Geometry: final body of the model. Coordinates: model frame, mm. A direction names the side the tool comes from. Round coordinates to 2 decimals unless told otherwise and drop trailing zeros. Loops run counter-clockwise (first coordinate to the right, second up) from the corner with the lowest first, then second, coordinate; pieces in that order, holes last. Notation, with made-up numbers: M -27,84.5 L 2,84.5 A11 cw 2,93.5 Z; hole C 49,73 d3. An arc over 180 degrees is marked long. Answer as a JSON object with one key per item and string values.
from build123d import *

# Parameters (mm, degrees)
F0_W     = 50.8
F0_H     = 76.2
F1_DEPTH = 101.6
F2_R     = 3.175
F3_W     = 6.770242
F3_H     = 4.11195
F4_DEPTH = 152.4


with BuildPart() as f1:
    # F0 (on Front) → F1 (new body)
    with BuildSketch(Plane.XZ):
        with Locations((25.4, 38.1)):
            Rectangle(F0_W, F0_H)
    extrude(amount=F1_DEPTH)

    # F2
    f2_edges = [f1.edges().sort_by_distance(p)[0] for p in [
        (50.8, -50.8, 76.2),
        (0, -50.8, 76.2),
        (25.4, 0, 76.2),
        (25.4, -101.6, 76.2),
        (0, -50.8, 0),
        (50.8, -50.8, 0),
        (25.4, 0, 0),
        (25.4, -101.6, 0),
    ]]
    fillet(f2_edges, radius=F2_R)

    # F3 (on face) → F4 (join)
    with BuildSketch(Plane.XY.offset(76.2)):
        with Locations((28.007837, -26.172377)):
            Rectangle(F3_W, F3_H)
    extrude(amount=F4_DEPTH)


solid = f1.part
1) Reachability of faces 1 (the flat face through (31.393, -26, 151)), 2 (the flat face through (28, -24.116, 151)), 3 (the flat face through (28, -28.228, 151)), 4 (the flat face through (24.623, -26, 151)) from +Z, -Z, +X, -X, +Y, -Y: full face, straight path, thin tool, end or side. Return the list, or none.
Results:
{"face 1": "+Z, +X, +Y, -Y", "face 2": "+Z, +X, -X, +Y", "face 3": "+Z, +X, -X, -Y", "face 4": "+Z, -X, +Y, -Y"}
2) Section query B-B (x = 15). Return the cut outline in (y, z) (3 decimals).
Results:
{"outline": "M -101.6,3.175 A3.175 ccw -98.425,0 L -3.175,0 A3.175 ccw 0,3.175 L 0,73.025 A3.175 ccw -3.175,76.2 L -98.425,76.2 A3.175 ccw -101.6,73.025 Z"}
3) Section query C-C (z = 142). Return the cut outline in (x, y), and give its area (3 significant figures).
Results:
{"outline": "M 24.62,-28.23 L 31.39,-28.23 L 31.39,-24.12 L 24.62,-24.12 Z", "area": "27.8 mm2"}
4) Ray query, line 1 (Z direction, x = 8.5, y = -95.5); line 2 (Y direction, x = 30.5, z = 84); line 3 (X direction, y = -54, z = 73.5). Return the intervals inside material, ascending.
Results:
{"line 1": "0 to 76.2", "line 2": "-28.23 to -24.12", "line 3": "0.04 to 50.76"}
5) Section query A-A (y = -73). Return the cut outline in (x, z) (3 decimals).
Results:
{"outline": "M 0,3.175 A3.175 ccw 3.175,0 L 47.625,0 A3.175 ccw 50.8,3.175 L 50.8,73.025 A3.175 ccw 47.625,76.2 L 3.175,76.2 A3.175 ccw 0,73.025 Z"}
6) Pin query (flat end, axial travel): P1, Ø7.5, axis at x = 29, z = 122, coming from the -Y side; P2, Ø8, axis at x = 21.5, z = 200.5, coming from the +Y side; P3, Ø1.2, axis at y = -26.5, z = 187.5, coming from the +X side. Return the tip coordinate at first contact, or that it passes through.
Results:
{"P1": "y = -28.23", "P2": "y = -24.12", "P3": "x = 31.39"}
7) Section query D-D (x = 28.5). Return the cut outline in (y, z) (3 decimals), and give its area (3 significant figures).
Results:
{"outline": "M -101.6,3.175 A3.175 ccw -98.425,0 L -3.175,0 A3.175 ccw 0,3.175 L 0,73.025 A3.175 ccw -3.175,76.2 L -24.116,76.2 L -24.116,228.6 L -28.228,228.6 L -28.228,76.2 L -98.425,76.2 A3.175 ccw -101.6,73.025 Z", "area": "8,360 mm2"}
